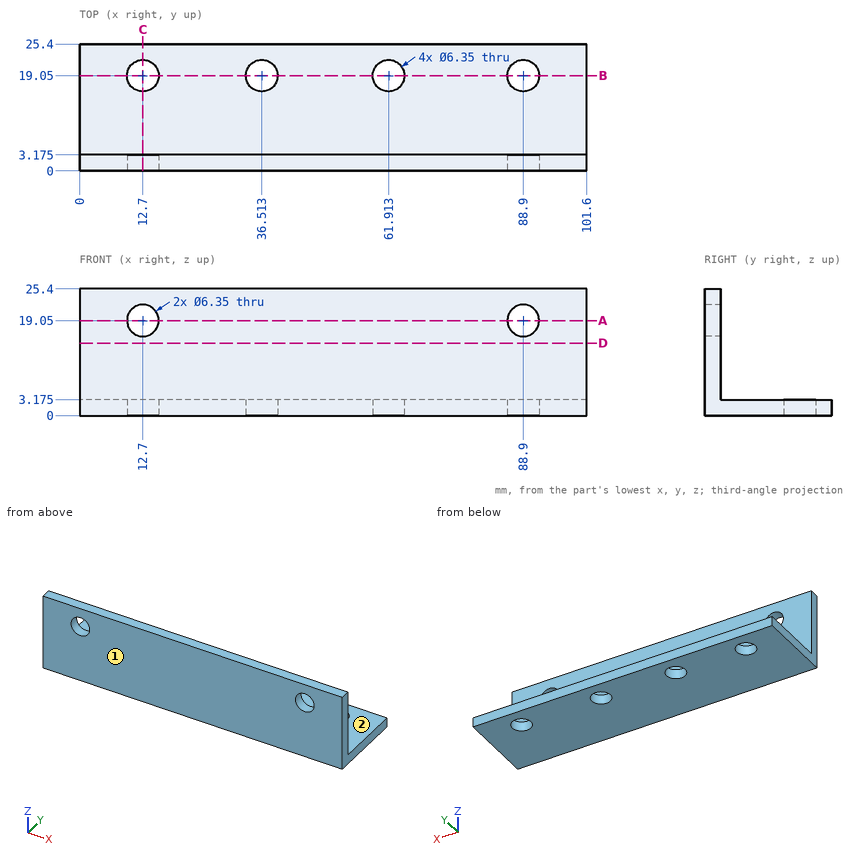
Study the drawing (mm; zero at the part's minimum x, y, z) and answer. A direction names the side the tool comes from. Coordinates: 2 decimals unless noted, no trailing zeros. Write each loop counter-clockwise with the first axis right and the second up, starting at its lowest first coordinate (ties: lowest second). Pieces come first, ordered by that corner, then holes. Notation, with made-up numbers: M 64.25,64.25 L 108.25,64.25 A4 ccw 108.25,70.25 Z; hole C 3,34 d6. An arc over 180 degrees is marked long. Use one line per item in the form item = value.
Item 1: Find section D-D, the plane z = 14.5. Give the vertices of the cut face in (x, y) (1 decimal).
Model answer:
outline = M 0,0 L 101.6,0 L 101.6,3.2 L 0,3.2 Z
Item 2: Find section B-B, the plane y = 19.05. Give the vertices of the cut face in (x, z) (1 decimal), plus the area to 3 significant figures.
Model answer:
outline = M 0,0 L 9.5,0 L 9.5,3.2 L 0,3.2 Z; M 15.9,0 L 33.3,0 L 33.3,3.2 L 15.9,3.2 Z; M 39.7,0 L 58.7,0 L 58.7,3.2 L 39.7,3.2 Z; M 65.1,0 L 85.7,0 L 85.7,3.2 L 65.1,3.2 Z; M 92.1,0 L 101.6,0 L 101.6,3.2 L 92.1,3.2 Z
area = 242 mm2
Item 3: Find section A-A, the plane z = 19.05. Give the vertices of the cut face in (x, y) (1 decimal).
Model answer:
outline = M 0,0 L 9.5,0 L 9.5,3.2 L 0,3.2 Z; M 15.9,0 L 85.7,0 L 85.7,3.2 L 15.9,3.2 Z; M 92.1,0 L 101.6,0 L 101.6,3.2 L 92.1,3.2 Z
Item 4: Find the intervals of material crossed by probe 1 along X at (y, z) = (19.05, 0.7) (1 decimal); probe 2 along Y at (x, z) = (88.9, 0.75) (1 decimal); probe 3 along Y at (x, z) = (40, 9.75) (1 decimal), in increasing order.
Model answer:
probe_1 = 0 to 9.5, 15.9 to 33.3, 39.7 to 58.7, 65.1 to 85.7, 92.1 to 101.6
probe_2 = 0 to 15.9, 22.2 to 25.4
probe_3 = 0 to 3.2
Item 5: For the marked faces 1 and 2, determine the directions among +Z, -Z, +X, -X, +Y, -Y from which every point of the face is accessible in a straight line to the end or side of a thin tool.
Model answer:
face_1 = +Z, -Z, +X, -X, -Y
face_2 = +Z, +X, -X, +Y
Item 6: Given P1, Ø8.5, axis at x = 36.51, y = 19.05, coming from the +Z side (1 decimal); P2, Ø1.5, axis at x = 89.5, z = 8.5, coming from the +Y side (1 decimal); P3, Ø5.5, axis at x = 88.9, y = 19.05, coming from the +Z side, each flat-ended and moving along its own axis, determine where each tip first touches the part or whether it passes through.
Model answer:
P1 = 3.2
P2 = 3.2
P3 = through
Item 7: Find section C-C, the plane x = 12.7. Give the vertices of the cut face in (y, z) (1 decimal), plus the area to 3 significant figures.
Model answer:
outline = M 0,0 L 15.9,0 L 15.9,3.2 L 3.2,3.2 L 3.2,15.9 L 0,15.9 Z; M 0,22.2 L 3.2,22.2 L 3.2,25.4 L 0,25.4 Z; M 22.2,0 L 25.4,0 L 25.4,3.2 L 22.2,3.2 Z
area = 111 mm2
